Design review of the part shown in the three views and the two pictorial views. Dimensions are in mm from the part's minimum x, y and z. A direction names the side the tool comes from. Give positions to 0.01 mm unless a question says otherwise; leave off trailing zeros. Loops run counter-clockwise (first coordinate to the right, second up) from the corner with the lowest first, then second, coordinate; pieces in that order, holes last. Notation, with made-up numbers: (-19.5, 64.25) - (-14.5, 64.25) arc R16 cw to (-14.5, 85.25) - close; hole circle Ø3 at (36, -14.75). An arc over 180 degrees is marked (long way). Use CSV: the item, a comma, the result in double quotes. Start each with the question number.
1. For pin 1 (10 mm diameter, centred on x = 25.5, z = 17, fed in from +Y); pin 2 (1.5 mm diameter, centred on x = 9, y = 21, fed in from -Z), all flat-tipped, find the tip position at first contact; note any pin that passes through.
2. Wall thickness on line 1 (X direction, y = 13.75, z = 22.5) (3 decimals); line 2 (Z direction, x = 3.5, y = 12); line 3 (X direction, y = 14.25, z = 23.25): over which ranges is each line inside the solid? List them lowest first.
3. Mouldability with a two-part tool opening along X and no side actions: class the marked faces 3, 4 and 5 as pulls with the +X half, pulls with the -X half, needs draft (parallel to the pull), parting line crosses it, or undercut.
4. Take a section at C-C on x = 15. Give the boundary of the cut face in (y, z).
5. For the marked faces 1 and 2, list the 3-axis set-ups (+Z, -Z, +X, -X, +Y, -Y) from which the entire face can be reached by the end or side of a thin tool; tool diameter is ignored.
6. Take a section at A-A on z = 4.5. Give the boundary of the cut face in (x, y), plus the area to 3 significant figures.
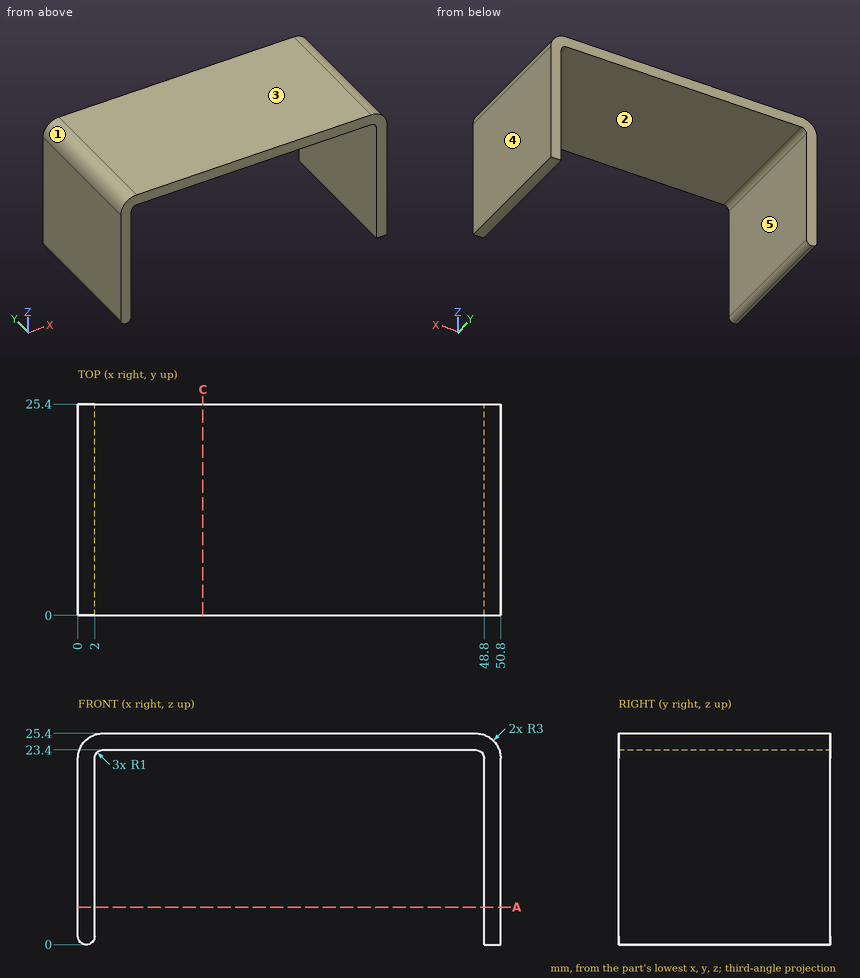
Check result:
1,pin 1,"passes through"
1,pin 2,"stops at z = 23.4"
2,line 1,"x = 0.002 to 2.005, 48.795 to 50.798"
2,line 2,"z = 23.4 to 25.4"
2,line 3,"x = 0.12 to 2.47, 48.33 to 50.68"
3,face 3,"needs draft"
3,face 4,"pulls with the +X half"
3,face 5,"undercut"
4,outline,"(0, 23.4) - (25.4, 23.4) - (25.4, 25.4) - (0, 25.4) - close"
5,face 1,"+Z, -X, +Y, -Y"
5,face 2,"-Z, +Y, -Y"
6,outline,"(0, 0) - (2, 0) - (2, 25.4) - (0, 25.4) - close; (48.8, 0) - (50.8, 0) - (50.8, 25.4) - (48.8, 25.4) - close"
6,area,"102 mm²"
